Here's how the part is built. I have some questions about the finished solid (model axes, mm). Face numbers are marked on the shaded views. Give positions to 0.01 mm unless a question says otherwise; leave off trailing zeros. Write each loop counter-clockwise with the first axis right and the second up, starting at its lowest first coordinate (ties: lowest second). Pieces come first, ordered by that corner, then holes. Notation, with made-up numbers: (35.5, 32) - (57.5, 32) arc R21 ccw to (57.5, 69) - close; hole circle Ø10 at (66.5, 79.25). An arc over 180 degrees is marked (long way). Write each question's results on one line, items separated by ' | '. Start each with the question number.
Item 1: Suppose I cut it at A-A on x = 0. List the corners of the cut face in (y, z) for me (3 decimals), then the cut area to 3 significant figures.
Item 2: Will these pins go through, and if not, where does the flat tip stop? P1, Ø4, axis at x = 65.66, z = 11.58, coming from the -Y side (3 decimals); P2, Ø2, axis at y = 1.5, z = 51, coming from the -X side; P3, Ø9, axis at x = -22.8, z = -62.65, coming from the +Y side; P4, Ø6, axis at y = 7.5, z = -39.5, coming from the -X side.
Item 3: Suppose I cut it at C-C on x = -16.5. List the corners of the cut face in (y, z) for me.
Item 4: Please list where these lines run through material, in increasing order: line 1 along Z through (x, y) = (-24.5, 11.75); line 2 along X through (y, z) = (9.25, 62.5); line 3 along Z through (x, y) = (-1, 5.5).
Item 5: We'd pull the mould along X, two halves only. Please class the marked faces 1, 2 and 3: +X half, -X half, draft (parallel to the pull), parting line (faces both ways), or undercut.
Item 6: Suppose I cut it at B-B on z = 0. List the corners of the cut face in (x, y) for me (3 decimals), then the cut area to 3 significant figures.
Autodesk Inventor part; units mm, degrees
ref_plane "Work Plane1" through (0, 0, -69.85) normal (0, 0, 1) x (1, 0, 0)
ref_plane "YZ Plane" through (0, 0, 0) normal (1, 0, 0) x (0, 1, 0)
ref_plane "XZ Plane" through (0, 0, 0) normal (0, 1, 0) x (-1, 0, 0)
sketch "Sketch1" plane through (0, 0, 0) normal (0, 1, 0) x (-1, 0, 0)
  circle A0 centre (0, 0) radius 57.15
  circle A1 centre (0, 0) radius 73.025
  dimension "d0" = 114.3
  dimension "d25" = 146.05
extrude "Extrusion1" add sketch "Sketch1" along normal blind 12.7
sketch "Sketch4" plane through (0, 12.7, 0) normal (0, 1, 0) x (1, 0, 0)
  line L0 (0, 0) -> (0, -66.675) construction
  line L1 (0, 0) -> (0, -57.15) construction
  circle A0 centre (0, 0) radius 57.15
  dimension "d14" = 66.675
  dimension "d33" = 0
hole "Hole2" at (0, 12.7, 66.675) direction (0, -1, 0) diameter 6.7564 end through all
pattern_circular "Circular Pattern2" count 18 over 360 about axis through (0, 0, 0) along (0, 1, 0) of "Hole2"
ref_plane "Work Plane1" through (0, 0, -69.85) normal (0, 0, 1) x (1, 0, 0)
properties part number "Injector Plate Retainer Ring" material "Aluminum 6061"
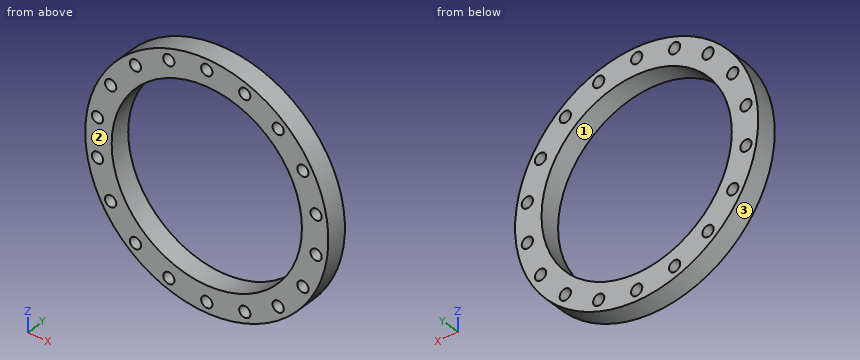
Checked values:
1) outline: (0, -73.025) - (12.7, -73.025) - (12.7, -70.053) - (0, -70.053) - close; (0, -63.297) - (12.7, -63.297) - (12.7, -57.15) - (0, -57.15) - close; (0, 57.15) - (12.7, 57.15) - (12.7, 63.297) - (0, 63.297) - close; (0, 70.053) - (12.7, 70.053) - (12.7, 73.025) - (0, 73.025) - close | area: 232 mm^2
2) P1: passes through | P2: stops at x = -53.22 | P3: stops at y = 12.7 | P4: stops at x = -63.25
3) outline: (0, -71.14) - (12.7, -71.14) - (12.7, -54.72) - (0, -54.72) - close; (0, 54.72) - (12.7, 54.72) - (12.7, 71.14) - (0, 71.14) - close
4) line 1: z = -68.79 to -65.58, -59.73 to -51.63, 51.63 to 59.73, 65.58 to 68.79 | line 2: x = -37.77 to -26.18, -19.43 to 19.43, 26.18 to 37.77 | line 3: z = -73.02 to -69.9, -63.45 to -57.14, 57.14 to 63.45, 69.9 to 73.02
5) face 1: undercut | face 2: draft | face 3: parting line
6) outline: (-73.025, 0) - (-57.15, 0) - (-57.15, 12.7) - (-73.025, 12.7) - close; (57.15, 0) - (73.025, 0) - (73.025, 12.7) - (57.15, 12.7) - close | area: 403 mm^2
